Input: part model. Units: mm. Frame: model coordinates. A direction names the side the tool comes from. Coordinates: 2 decimals unless noted, no trailing zeros. Loops run counter-clockwise (first coordinate to the right, second up) from the corner with the lowest first, then second, coordinate; pieces in that order, holes last.
(1) Section D-D, the plane z = -1.25. Return loops of the section in (x, y).
(2) Mould query, pull axis Z, two halves, no side actions, for faces 1 (the face through (16.563, 3.525, -9.452)), 2 (the face through (-16, 2, -4.762)), 3 (the face through (19.05, 2, 1)). Classes: released by +Z, released by -Z, zero draft, split by the parting line, or undercut.
(3) Section C-C, the plane y = 0.75. Return loops of the section in (x, z), then the cut area to 3 significant figures.
(4) Set-up query: faces 4 (the face through (6, 2, -4.762)), 5 (the face through (0, 3.048, 1)), 6 (the face through (0, 0, 0)). Return all of +Z, -Z, +X, -X, +Y, -Y with unobstructed straight access to the full face (end or side cutting, diameter ignored); none if empty.
(5) Section A-A, the plane y = 3.75. Return loops of the section in (x, z), then the cut area to 3 significant figures.
(6) Line query: L1, parallel to X at y = 5.5, z = -6.25; L2, parallel to Z at x = -12, y = 3; L3, parallel to Y at x = 7.5, z = 2.5. Output: solid intervals per line, ascending.
(7) Contact query for flat-ended pins moving along their axis: P1, Ø1.5, axis at x = -17.5, y = 1, coming from the -Z side; P2, Ø4, axis at x = -4, z = 3, coming from the +Y side; P3, Ø2, axis at y = 5, z = -5, coming from the -X side. Output: stop coordinate, or through.
```python
from build123d import *

# Parameters (mm, degrees)
SKETCH1_W                    = 38.1
SKETCH1_H                    = 15.875
BOSS_EXTRUDE1_DEPTH          = 3.048
SKETCH2_R                    = 3.175
BOSS_EXTRUDE2_DEPTH          = 1.27
BOSS_EXTRUDE2_DEPTH_BACK     = 39.37
SKETCH7_W                    = 12.7
SKETCH7_H                    = 6.35
CUT_EXTRUDE_THIN2_DEPTH      = 7.223
CUT_EXTRUDE_THIN2_DEPTH_BACK = 1.127
SKETCH8_R                    = 1.5875
CUT_EXTRUDE2_DEPTH           = 40.37
SKETCH9_R                    = 1.524
CUT_EXTRUDE3_DEPTH           = 4.175


with BuildPart() as part:
    # Sketch1 → Boss-Extrude1 (new body)
    with BuildSketch(Plane(origin=(0, 0, 0), x_dir=(1, 0, 0), z_dir=(0, 1, 0))):
        Rectangle(SKETCH1_W, SKETCH1_H)
    extrude(amount=BOSS_EXTRUDE1_DEPTH)

    # Sketch2 → Boss-Extrude2 (add, two sides)
    with BuildSketch(Plane(origin=(19.05, 0, 0), x_dir=(0, 0, -1), z_dir=(1, 0, 0))) as boss_extrude2_sk:
        with Locations((7.9375, 3.048)):
            Circle(SKETCH2_R)
    extrude(amount=BOSS_EXTRUDE2_DEPTH)
    extrude(boss_extrude2_sk.sketch, amount=-BOSS_EXTRUDE2_DEPTH_BACK)

    # Sketch7 → Cut-Extrude-Thin2 (cut, two sides)
    with BuildSketch(Plane(origin=(0, 0, 0), x_dir=(1, 0, 0), z_dir=(0, 1, 0))) as cut_extrude_thin2_sk:
        with Locations((-19.05, 7.9375)):
            Rectangle(SKETCH7_W, SKETCH7_H)
        with Locations((6.35, 7.9375)):
            Rectangle(SKETCH7_W, SKETCH7_H)
    extrude(amount=CUT_EXTRUDE_THIN2_DEPTH, mode=Mode.SUBTRACT)
    extrude(cut_extrude_thin2_sk.sketch, amount=-CUT_EXTRUDE_THIN2_DEPTH_BACK, mode=Mode.SUBTRACT)

    # Sketch8 → Cut-Extrude2 (cut, through all)
    with BuildSketch(Plane(origin=(20.32, 0, 0), x_dir=(0, 0, -1), z_dir=(1, 0, 0))):
        with Locations((7.9375, 3.048)):
            Circle(SKETCH8_R)
    extrude(amount=-CUT_EXTRUDE2_DEPTH, mode=Mode.SUBTRACT)

    # Sketch9 → Cut-Extrude3 (cut, through all)
    with BuildSketch(Plane(origin=(0, 3.048, 0), x_dir=(1, 0, 0), z_dir=(0, 1, 0))):
        with Locations((-12.7, -1.5875)):
            Circle(SKETCH9_R)
        with Locations((12.7, -1.5875)):
            Circle(SKETCH9_R)
    extrude(amount=-CUT_EXTRUDE3_DEPTH, mode=Mode.SUBTRACT)


solid = part.part
```
Report:
1. outline: (-19.05, 0) - (19.05, 0) - (19.05, 3.05) - (-19.05, 3.05) - close
2. face 1: undercut
2. face 2: released by -Z
2. face 3: zero draft
3. outline: (-19.05, -4.76) - (-12.7, -4.76) - (-12.7, -10.13) - (0, -10.13) - (0, -4.76) - (12.7, -4.76) - (12.7, -10.13) - (20.32, -10.13) - (20.32, -5.75) - (19.05, -5.75) - (19.05, 7.94) - (-19.05, 7.94) - close; hole circle Ø3.05 at (-12.7, 1.59); hole circle Ø3.05 at (12.7, 1.59)
3. area: 577 mm2
4. face 4: -Z, +Y, -Y
4. face 5: +Z, +X, -X, +Y
4. face 6: +Z, +X, -X, -Y
5. outline: (-12.7, -11.03) - (0, -11.03) - (0, -9.36) - (-12.7, -9.36) - close; (-12.7, -6.51) - (0, -6.51) - (0, -4.84) - (-12.7, -4.84) - close; (12.7, -11.03) - (20.32, -11.03) - (20.32, -9.36) - (12.7, -9.36) - close; (12.7, -6.51) - (20.32, -6.51) - (20.32, -4.84) - (12.7, -4.84) - close
5. area: 68.0 mm2
6. L1: x = -12.7 to 0, 12.7 to 20.32
6. L2: z = -11.11 to -9.52, -6.35 to 0.23, 2.94 to 7.94
6. L3: y = 0 to 3.05
7. P1: stops at z = -4.76
7. P2: stops at y = 3.05
7. P3: stops at x = -12.7
